The listing builds one solid part. Answer for the finished solid, in the listing's coordinates (mm). A direction names the side the tool comes from. Coordinates: 2 decimals unless noted, no trailing zeros. Order: outer loops, then holes, each group sorted by start corner. A loop starts at its lowest first (then second) coordinate and runs counter-clockwise, first axis right, second up. Notation, with made-up numbers: (44, -17) - (60, -17) arc R15 cw to (60, 4) - close; hole circle Ø8 at (37, -33). An arc over 180 degrees is marked (long way). Use one line per item in the form item = value. Start each with the question number.
Item 1: Section A-A, the plane x = -38.5 is taken. Write down the section's boundary in (y, z), and give its area (3 significant figures).
Item 2: Section D-D, the plane x = -48.5 is taken. Write down the section's boundary in (y, z).
Item 3: A tool of negligible diameter and unlimited length cuts with its end or side. For faces 1 (the flat face through (-45.12, 25.14, 1.48)), 2 (the flat face through (-56.674, 18.616, 1.479)), from which of +Z, -Z, +X, -X, +Y, -Y can it reach the whole face along a straight path? Write none if from no direction.
Item 4: Section C-C, the plane x = -61 is taken. Write down the section's boundary in (y, z).
Item 5: Consider line 1 along Y through (x, z) = (-68, 1.75); line 2 along X through (y, z) = (34, 2.85); line 3 along X through (y, z) = (26, 1.35). Determine where each line is inside the solid, lowest interval first. Write a range as [from, to].
Item 6: The mould has two halves that part along X. Classify faces 3 (the cylindrical face through (-25.141, 35.707, 1.479)), 4 (the cylindrical face through (-37.73, 21.35, 1.48)), 5 (the flat face through (-52.23, 4.46, 1.48)): released by +X, released by -X, zero draft, split by the parting line, or undercut.
Item 7: Section B-B, the plane z = 0.65 is taken. Count the separate pieces of the cut face and the enclosed holes in it, and give its area (3 significant figures).
from build123d import *

# Parameters (mm, degrees)
SKETCH1_R       = 1
SKETCH1_R_2     = 3.5
SKETCH1_R_3     = 0.952573724
SKETCH1_R_4     = 0.980307261
EXTRUDE_6_DEPTH = 3


with BuildPart() as part:
    # Sketch1 → Бобышка-Вытянуть6 (new body)
    with BuildSketch(Plane.XY):
        with BuildLine():
            Line((-50.090575528, 20.246358773), (-63.443383911, 16.939772721))
            Line((-63.443383911, 16.939772721), (-64.348156071, 17.355557159))
            ThreePointArc((-64.348156071, 17.355557159), (-76.371742075, 7.335892912), (-61.608311767, 2.139604087))
            Line((-61.608311767, 2.139604087), (-42.594837437, 6.847953613))
            Line((-42.594837437, 6.847953613), (-28.633720832, 20.587239783))
            ThreePointArc((-28.633720832, 20.587239783), (-25.336971544, 35.887296519), (-40.166847554, 30.883790793))
            Line((-40.166847554, 30.883790793), (-40.285943738, 29.895203185))
            Line((-40.285943738, 29.895203185), (-50.090575528, 20.246358773))
        make_face()
        with Locations((-27.098820281, 33.552896146)):
            Circle(SKETCH1_R, mode=Mode.SUBTRACT)
        with Locations((-67.514190904, 8.930818383)):
            Circle(SKETCH1_R_2, mode=Mode.SUBTRACT)
        with Locations((-60.675780867, 10.535905116)):
            Circle(SKETCH1_R, mode=Mode.SUBTRACT)
        with Locations((-66.377650396, 3.14132137)):
            Circle(SKETCH1_R, mode=Mode.SUBTRACT)
        with Locations((-68.59259333, 14.731425956)):
            Circle(SKETCH1_R, mode=Mode.SUBTRACT)
        with Locations((-57.675780867, 11.227745586)):
            Circle(SKETCH1_R_3, mode=Mode.SUBTRACT)
        with Locations((-54.753543693, 11.906369118)):
            Circle(SKETCH1_R_4, mode=Mode.SUBTRACT)
        with Locations(Location((-40.543510307, 19.856172639, 0), (0, 0, 180))):
            Circle(SKETCH1_R_4, mode=Mode.SUBTRACT)
        with Locations(Location((-38.436147278, 21.991359062, 0), (0, 0, 180))):
            Circle(SKETCH1_R_3, mode=Mode.SUBTRACT)
        with Locations(Location((-35.709722432, 33.127748875, 0), (0, 0, 180))):
            Circle(SKETCH1_R, mode=Mode.SUBTRACT)
        with Locations(Location((-26.991820916, 25.175724624, 0), (0, 0, 180))):
            Circle(SKETCH1_R, mode=Mode.SUBTRACT)
        with Locations(Location((-36.27683183, 24.185897745, 0), (0, 0, 180))):
            Circle(SKETCH1_R, mode=Mode.SUBTRACT)
        with Locations(Location((-73.460528059, 7.615837609, 0), (0, 0, 180))):
            Circle(SKETCH1_R, mode=Mode.SUBTRACT)
        with Locations(Location((-31.330827271, 29.173602043, 0), (0, 0, 180))):
            Circle(SKETCH1_R_2, mode=Mode.SUBTRACT)
    extrude(amount=EXTRUDE_6_DEPTH)


solid = part.part
Response:
q1.outline = (10.88, 0) - (21.04, 0) - (21.04, 3) - (10.88, 3) - close; (22.94, 0) - (34.61, 0) - (34.61, 3) - (22.94, 3) - close
q1.area = 65.5 mm2
q2.outline = (5.39, 0) - (21.81, 0) - (21.81, 3) - (5.39, 3) - close
q3.face_1 = +Z, -Z, -X, +Y
q3.face_2 = +Z, -Z, +Y
q4.outline = (2.29, 0) - (9.59, 0) - (9.59, 3) - (2.29, 3) - close; (11.48, 0) - (17.54, 0) - (17.54, 3) - (11.48, 3) - close
q5.line_1 = [-0.06, 5.46], [12.4, 13.93], [15.54, 17.92]
q5.line_2 = [-38.93, -36.2], [-35.22, -27.99], [-26.2, -23.73]
q5.line_3 = [-44.24, -32.81], [-29.85, -27.56], [-26.43, -22.91]
q6.face_3 = split by the parting line
q6.face_4 = undercut
q6.face_5 = released by +X
q7.separate_pieces = 1
q7.enclosed_holes = 14
q7.area = 805 mm2
